For this review, take the finished solid that the model builds, in its own axes (mm). A direction names the side the tool comes from. Coordinates: 2 decimals unless noted, no trailing zeros. Order: outer loops, then holes, each group sorted by start corner. A loop starts at its lowest first (then second) coordinate and runs counter-clockwise, first axis right, second up. Notation, with made-up numbers: (5.5, 41.25) -> (19.5, 41.25) arc R13 cw to (19.5, 51.25) -> close; hole circle Ø2 at (69.5, 35.5). An arc over 180 degrees is marked (long way). Answer as a JSON object with one key per item and string values. Group by question number.
1) Add section C-C, the plane x = 8. Write out the cut boundary in (y, z), then the cut area to 3 significant figures.
2) For pin 1 (1.5 mm diameter, centred on x = 8, z = -0.5, fed in from -Y), flat-tipped, find the tip position at first contact; note if it passes through.
3) Add section B-B, the plane z = 0. Write out the cut boundary in (x, y).
4) Machinability: for faces 3 (the cylindrical face through (10, 58, 0)), 4 (the cylindrical face through (0, 27, 2)), 5 (the flat face through (0, 0, 0)), which of the approach directions +Z, -Z, +X, -X, +Y, -Y give a long, thin tool a straight path to every point of the face, cutting with its end or side? Answer none if there is none.
5) Draft analysis for pull direction X (two halves, no side actions). For faces 1 (the flat face through (19, 0, 0)), 2 (the cylindrical face through (20.6, 26.1, 1.2)), state which applies: +X half, -X half, draft (parallel to the pull), parting line (faces both ways), or undercut.
6) Add section A-A, the plane y = 48. Write out the cut boundary in (x, z).
7) Wall thickness on L1, parallel to X at y = 47, z = 0.15; L2, parallel to X at y = 20, z = 1.5; L3, parallel to Y at x = 5.5, z = -0.15: over which ranges is each line inside the solid? List them lowest first.
from build123d import *

# Parameters (mm, degrees)
ESQUISSE2_R = 2


with BuildPart() as part:
    # Balayage1: sweep along a path in Esquisse1
    with BuildLine(Plane.XY) as balayage1_path:
        Line((0, 0), (0, 53))
        ThreePointArc((0, 53), (0.878679656, 55.121320344), (3, 56))
        Line((3, 56), (16, 56))
        ThreePointArc((16, 56), (18.121320344, 55.121320344), (19, 53))
        Line((19, 53), (19, 0))
    # Esquisse2 → Balayage1 (sweep)
    with BuildSketch(Plane(origin=(0, 0, 0), x_dir=(1, 0, 0), z_dir=(0, 1, 0))):
        Circle(ESQUISSE2_R)
    sweep(path=balayage1_path.line)


solid = part.part
Output values:
{
 "1": {"outline": "circle Ø4 at (56, 0)", "area": "12.6 mm²"},
 "2": {"pin 1": "stops at y = 54"},
 "3": {"outline": "(-2, 0) -> (2, 0) -> (2, 53) arc R1 cw to (3, 54) -> (16, 54) arc R1 cw to (17, 53) -> (17, 0) -> (21, 0) -> (21, 53) arc R5 ccw to (16, 58) -> (3, 58) arc R5 ccw to (-2, 53) -> close"},
 "4": {"face 3": "none", "face 4": "-Y", "face 5": "+Z, -Z, +X, -X, -Y"},
 "5": {"face 1": "draft", "face 2": "undercut"},
 "6": {"outline": "circle Ø4 at (0, 0); circle Ø4 at (19, 0)"},
 "7": {"L1": "x = -1.99 to 1.99, 17.01 to 20.99", "L2": "x = -1.32 to 1.32, 17.68 to 20.32", "L3": "y = 54.01 to 57.99"}
}
